CAD build for the part. Positions are in the model's coordinates, mm. Face numbers are marked on the shaded views. Coordinates: 2 decimals unless noted, no trailing zeros. Loops run counter-clockwise (first coordinate to the right, second up) from the corner with the lowest first, then second, coordinate; pieces in that order, holes last.
1) Saw through at B-B, the plane x = -27.5. Write the cut outline in (y, z).
2) Saw through at C-C, the plane y = -6.5. Write the cut outline in (x, z), and give its area (3 significant figures).
3) Wall check: line 1 along X through (y, z) = (-11, 0.5); line 2 along Y through (x, z) = (-27.5, -7.5); line 3 along X through (y, z) = (2.5, 1.5). Give the ranges that are in metal, low to high.
4) Saw through at D-D, the plane y = 0. Write the cut outline in (x, z), and give its area (3 significant figures).
5) Two-plate mould, pull along X, no slides. Class the marked faces 1, 2, 3 and 4: +X half, -X half, draft (parallel to the pull), parting line (faces both ways), or undercut.
6) Saw through at A-A, the plane z = 0. Write the cut outline in (x, y), and give its area (3 significant figures).
7) Pin check, flat tips, straight feed: pin 1 Ø5.5 at (x, y) = (-27.5, 0) entering from -Z; pin 2 Ø9 at (x, z) = (-27.5, 0) entering from +Y. Stop position of each tip, or through.
```python
from build123d import *

# Parameters (mm, degrees)
F0_W     = 80
F0_H     = 25
F0_R     = 5
F1_DEPTH = 15
F3_D     = 4.2
F3_DEPTH = 14.4
F3_TIP   = 1.2618073


with BuildPart() as f1:
    # F0 (on Front) → F1 (new body, symmetric)
    with BuildSketch(Plane.XZ):
        Rectangle(F0_W, F0_H)
        with Locations((-27.5, 0)):
            Circle(F0_R, mode=Mode.SUBTRACT)
        with Locations((27.5, 0)):
            Circle(F0_R, mode=Mode.SUBTRACT)
    extrude(amount=F1_DEPTH, both=True)

    # F3
    with Locations(Plane(origin=(0, 0, -12.5), x_dir=(1, 0, 0), z_dir=(0, 0, -1))):
        with Locations((-27.5, 0), (27.5, 0)):
            Hole(F3_D / 2, depth=F3_DEPTH)
            with Locations((0, 0, -(F3_DEPTH + F3_TIP / 2))):  # 118° drill point
                Cone(0, F3_D / 2, F3_TIP, mode=Mode.SUBTRACT)


solid = f1.part
```
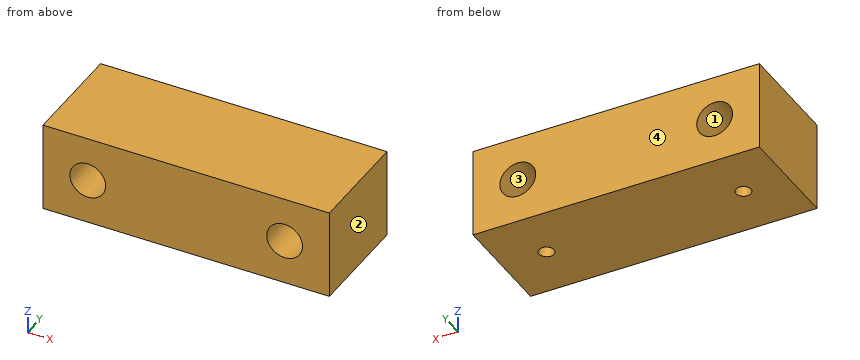
Data:
1. outline: (-15, -12.5) - (-2.1, -12.5) - (-2.1, -5) - (-15, -5) - close; (-15, 5) - (15, 5) - (15, 12.5) - (-15, 12.5) - close; (2.1, -12.5) - (15, -12.5) - (15, -5) - (2.1, -5) - close
2. outline: (-40, -12.5) - (40, -12.5) - (40, 12.5) - (-40, 12.5) - close; hole circle Ø10 at (-27.5, 0); hole circle Ø10 at (27.5, 0)
2. area: 1,840 mm2
3. line 1: x = -40 to -32.47, -22.53 to 22.53, 32.47 to 40
3. line 2: y = -15 to -2.1, 2.1 to 15
3. line 3: x = -40 to -32.27, -22.73 to 22.73, 32.27 to 40
4. outline: (-40, -12.5) - (-29.6, -12.5) - (-29.6, -4.54) arc R5 cw (long way) to (-25.4, -4.54) - (-25.4, -12.5) - (25.4, -12.5) - (25.4, -4.54) arc R5 cw (long way) to (29.6, -4.54) - (29.6, -12.5) - (40, -12.5) - (40, 12.5) - (-40, 12.5) - close
4. area: 1,780 mm2
5. face 1: undercut
5. face 2: +X half
5. face 3: undercut
5. face 4: draft
6. outline: (-40, -15) - (-32.5, -15) - (-32.5, 15) - (-40, 15) - close; (-22.5, -15) - (22.5, -15) - (22.5, 15) - (-22.5, 15) - close; (32.5, -15) - (40, -15) - (40, 15) - (32.5, 15) - close
6. area: 1,800 mm2
7. pin 1: stops at z = -12.5
7. pin 2: passes through
